Drawing for the job (mm, zero at the part's lowest x, y, z). Coordinates: 2 decimals unless noted, no trailing zeros. Write each loop counter-clockwise with the first axis right and the second up, starting at its lowest first coordinate (ties: lowest second). Pieces come first, ordered by that corner, then holes. Notation, with made-up numbers: (26.25, 80) - (73.25, 80) arc R28 ccw to (73.25, 107) - close; hole circle Ø4 at (-17, -3). An arc over 180 degrees is marked (long way). Write each question's results on one line, items separated by ' | '.
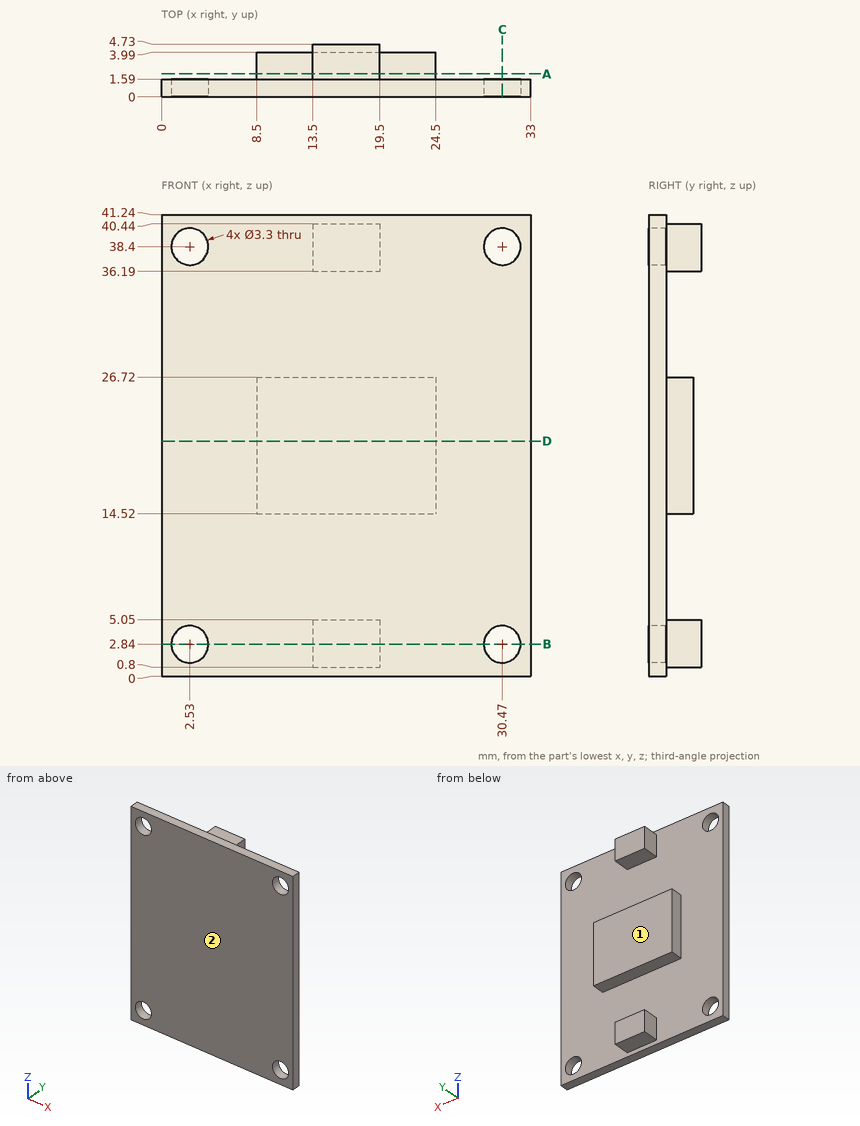
(1) Saw through at D-D on z = 21. Write the cut outline in (x, y).
Return value:
outline: (0, 0) - (33, 0) - (33, 1.59) - (24.5, 1.59) - (24.5, 3.99) - (8.5, 3.99) - (8.5, 1.59) - (0, 1.59) - close
(2) Two-plate mould, pull along Z, no slides. Class the marked faces 1 and 2: released by +Z, released by -Z, zero draft, split by the parting line, or undercut.
Return value:
face 1: undercut | face 2: zero draft
(3) Saw through at A-A on y = 2.05. Write the cut outline in (x, z).
Return value:
outline: (8.5, 14.52) - (24.5, 14.52) - (24.5, 26.72) - (8.5, 26.72) - close; (13.5, 0.8) - (19.5, 0.8) - (19.5, 5.05) - (13.5, 5.05) - close; (13.5, 36.19) - (19.5, 36.19) - (19.5, 40.44) - (13.5, 40.44) - close
(4) Flat gauge pins, fed straight in: P1, Ø1.2, axis at x = 20, y = 2.5, coming from the -Z side; P2, Ø4, axis at x = 21.5, z = 20.5, coming from the +Y side; P3, Ø2, axis at y = 3.5, z = 24.5, coming from the -X side; P4, Ø2, axis at x = 2.53, z = 38.4, coming from the -Y side. Where does each tip first touch, or does it go through?
Return value:
P1: stops at z = 0.8 | P2: stops at y = 3.99 | P3: stops at x = 8.5 | P4: passes through
(5) Saw through at C-C on x = 30.47. Write the cut outline in (y, z).
Return value:
outline: (0, 0) - (1.59, 0) - (1.59, 1.19) - (0, 1.19) - close; (0, 4.49) - (1.59, 4.49) - (1.59, 36.75) - (0, 36.75) - close; (0, 40.05) - (1.59, 40.05) - (1.59, 41.24) - (0, 41.24) - close
(6) Saw through at B-B on z = 2.84. Write the cut outline in (x, y).
Return value:
outline: (0, 0) - (0.88, 0) - (0.88, 1.59) - (0, 1.59) - close; (4.18, 0) - (28.82, 0) - (28.82, 1.59) - (19.5, 1.59) - (19.5, 4.73) - (13.5, 4.73) - (13.5, 1.59) - (4.18, 1.59) - close; (32.12, 0) - (33, 0) - (33, 1.59) - (32.12, 1.59) - close
(7) Wall check: line 1 (Z direction, x = 30.47, y = 1.2); line 2 (X direction, y = 1.2, z = 2.84); line 3 (Z direction, x = 16, y = 3.85). Give the ranges that are in metal, low to high. Write a range as from..to.
Return value:
line 1: z = 0..1.19, 4.49..36.75, 40.05..41.24 | line 2: x = 0..0.88, 4.18..28.82, 32.12..33 | line 3: z = 0.8..5.05, 14.52..26.72, 36.19..40.44
